```python
from build123d import *

# Parameters (mm, degrees)
BOSS_EXTRUDE1_DEPTH   = 1.6
SKETCH2_R             = 3.45
BOSS_EXTRUDE2_DEPTH   = 1.4
M6X1_0_TAPPED_HOLE1_D = 5


with BuildPart() as part:
    # Sketch1 → Boss-Extrude1 (new body)
    with BuildSketch(Plane.XY):
        with BuildLine():
            Line((-6.237396753, 4.481095129), (-3, 5))
            Line((-3, 5), (3, 5))
            Line((3, 5), (6.237396753, 4.481095129))
            ThreePointArc((6.237396753, 4.481095129), (7.141511088, 3.973114811), (7.5, 3))
            Line((7.5, 3), (7.5, -3))
            ThreePointArc((7.5, -3), (7.141511088, -3.973114811), (6.237396753, -4.481095129))
            Line((6.237396753, -4.481095129), (3, -5))
            Line((3, -5), (-3, -5))
            Line((-3, -5), (-6.237396753, -4.481095129))
            ThreePointArc((-6.237396753, -4.481095129), (-7.141511088, -3.973114811), (-7.5, -3))
            Line((-7.5, -3), (-7.5, 3))
            ThreePointArc((-7.5, 3), (-7.141511088, 3.973114811), (-6.237396753, 4.481095129))
        make_face()
    extrude(amount=BOSS_EXTRUDE1_DEPTH)

    # Sketch2 → Boss-Extrude2 (add)
    with BuildSketch(Plane.XY.offset(1.6)):
        Circle(SKETCH2_R)
    extrude(amount=BOSS_EXTRUDE2_DEPTH)

    # M6x1.0 Tapped Hole1 (through all)
    with Locations(Plane.XY.offset(3)):
        with Locations((0, 0)):
            Hole(M6X1_0_TAPPED_HOLE1_D / 2)


solid = part.part
```
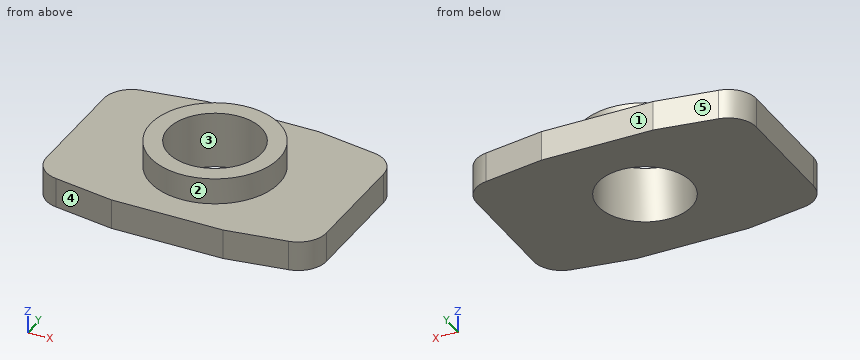
Geometry check sheet. Reference: the model listing, model coordinates, mm. Face numbers are marked on the shaded views. A direction names the side the tool comes from. Give positions to 0.01 mm unless a question says otherwise; leave off trailing zeros. Write each loop counter-clockwise with the first axis right and the second up, starting at its lowest first coordinate (ties: lowest second). Pieces come first, ordered by that corner, then holes.
1) Section check C-C, the plane z = 1.1. Record the boundary of the cut face in (x, y).
2) Section check A-A, the plane x = 0. Record the boundary of the cut face in (y, z).
3) Access from +Z, -Z, +X, -X, +Y, -Y to the whole of each face (thin tool, end or side, straight path). Record for the marked faces 1 and 2.
4) Section check B-B, the plane y = 0. Record the boundary of the cut face in (x, z), and give its area (3 significant figures).
5) Material ranges on L1, parallel to Y at x = 0, z = 2.2; L2, parallel to Y at x = 0, z = 1.3; L3, parallel to Z at x = -4.25, y = -0.75, recorded low to high.
6) Section check D-D, the plane z = 1.9. Record the boundary of the cut face in (x, y), and give its area (3 significant figures).
7) Release check for a two-part mould opening along Y. For the marked faces 3, 4 and 5 record: pulls with the +Y half, pulls with the -Y half, needs draft (parallel to the pull), parting line crosses it, or undercut.
8) Gauge pin test, flat ends, axial feed: pin 1 (1 mm diameter, centred on x = 5.5, z = 2, fed in from -Y); pin 2 (2 mm diameter, centred on x = 4.5, y = -3.5, fed in from +Z). Record the tip position at first contact, or that the pin passes through.
Computed:
1. outline: (-7.5, -3) arc R1.5 ccw to (-6.24, -4.48) - (-3, -5) - (3, -5) - (6.24, -4.48) arc R1.5 ccw to (7.5, -3) - (7.5, 3) arc R1.5 ccw to (6.24, 4.48) - (3, 5) - (-3, 5) - (-6.24, 4.48) arc R1.5 ccw to (-7.5, 3) - close; hole circle Ø5 at (0, 0)
2. outline: (-5, 0) - (-2.5, 0) - (-2.5, 3) - (-3.45, 3) - (-3.45, 1.6) - (-5, 1.6) - close; (2.5, 0) - (5, 0) - (5, 1.6) - (3.45, 1.6) - (3.45, 3) - (2.5, 3) - close
3. face 1: +Z, -Z, +X, -X, +Y
3. face 2: +Z
4. outline: (-7.5, 0) - (-2.5, 0) - (-2.5, 3) - (-3.45, 3) - (-3.45, 1.6) - (-7.5, 1.6) - close; (2.5, 0) - (7.5, 0) - (7.5, 1.6) - (3.45, 1.6) - (3.45, 3) - (2.5, 3) - close
4. area: 18.7 mm2
5. L1: y = -3.45 to -2.5, 2.5 to 3.45
5. L2: y = -5 to -2.5, 2.5 to 5
5. L3: z = 0 to 1.6
6. outline: circle Ø6.9 at (0, 0); hole circle Ø5 at (0, 0)
6. area: 17.8 mm2
7. face 3: undercut
7. face 4: pulls with the -Y half
7. face 5: pulls with the +Y half
8. pin 1: stops at y = -4.65
8. pin 2: stops at z = 1.6
